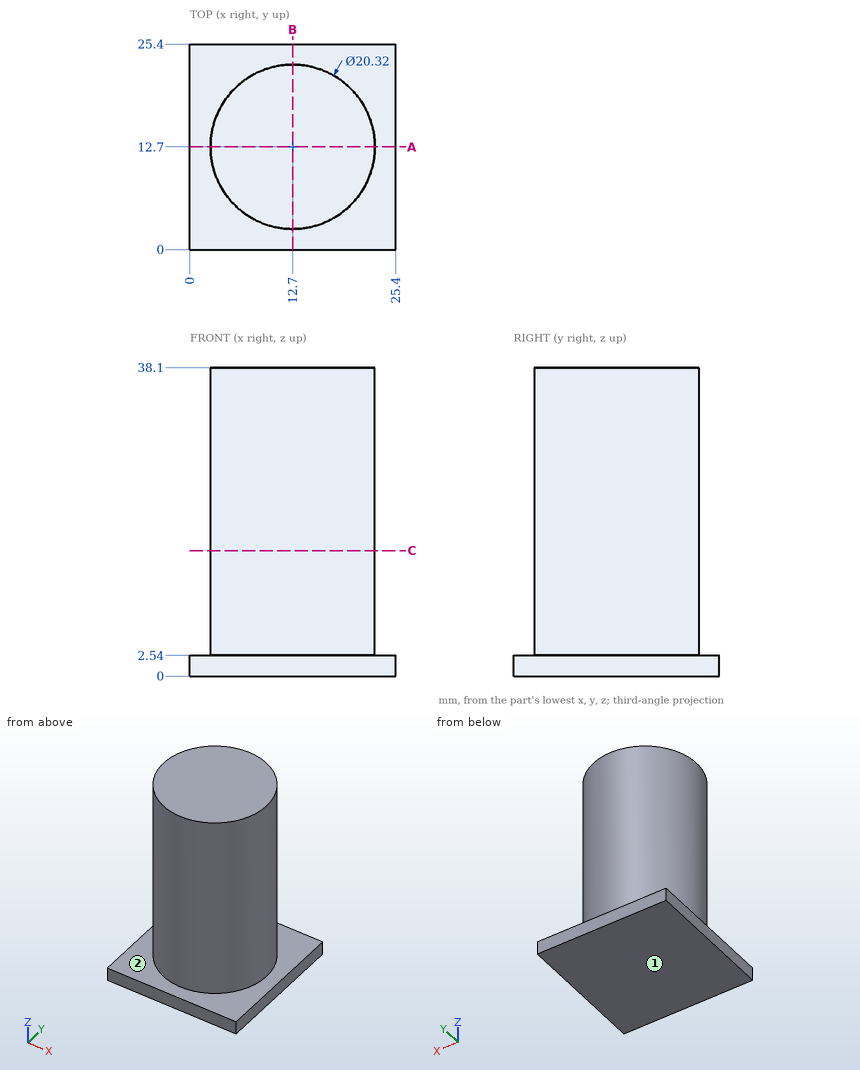
Can you work these out from the drawing? Everything is in mm from the part's minimum corner. A direction names the side the tool comes from. Coordinates: 2 decimals unless noted, no trailing zeros. Write each loop counter-clockwise with the first axis right and the second up, starting at its lowest first coordinate (ties: lowest second). Pieces come first, ordered by that corner, then holes. Notation, with made-up numbers: (54, 7) -> (103, 7) arc R5 cw to (103, 12) -> close; hole circle Ø7 at (57, 1.5). An arc over 180 degrees is marked (long way). Return JSON: item names as keys, results as strings.
(1) I need wall thicknesses on L1, parallel to Y at x = 12.75, z = 15.5; L2, parallel to Z at x = 23, y = 14.25; L3, parallel to Y at x = 6.25, z = 36. Which ranges of each line are inside material? Lowest first, please.
Numbers:
{"L1": "y = 2.54 to 22.86", "L2": "z = 0 to 2.54", "L3": "y = 4.85 to 20.55"}
(2) Imagine slicing it at A-A, the plane y = 12.7. Please give me the cut outline in (x, z), then the cut area to 3 significant figures.
Numbers:
{"outline": "(0, 0) -> (25.4, 0) -> (25.4, 2.54) -> (22.86, 2.54) -> (22.86, 38.1) -> (2.54, 38.1) -> (2.54, 2.54) -> (0, 2.54) -> close", "area": "787 mm2"}
(3) I'm going to push flat-ended pins straight in: pin 1 (8 mm diameter, centred on y = 3.5, z = 16, fed in from +X); pin 2 (3 mm diameter, centred on y = 21.5, z = 25, fed in from +X); pin 3 (2 mm diameter, centred on y = 4, z = 34, fed in from -X). Where does each tip first touch, or does it pass through?
Numbers:
{"pin 1": "stops at x = 21.43", "pin 2": "stops at x = 19.77", "pin 3": "stops at x = 6.07"}
(4) Imagine slicing it at C-C, the plane z = 15.5. Please give me the cut outline in (x, y).
Numbers:
{"outline": "circle Ø20.32 at (12.7, 12.7)"}
(5) Which directions (+Z, -Z, +X, -X, +Y, -Y) give clear straight access to the entire face, cutting with the end or side of a thin tool? Please do the marked faces 1 and 2.
Numbers:
{"face 1": "-Z, +X, -X, +Y, -Y", "face 2": "+Z"}
